The listing builds one solid part. Answer for the finished solid, in the listing's coordinates (mm). Coordinates: 2 decimals unless noted, no trailing zeros. Loops run counter-clockwise (first coordinate to the right, second up) from the corner with the lowest first, then second, coordinate; pieces in that order, holes last. Notation, with made-up numbers: M 24.25,78.25 L 55.25,78.25 A29 cw 55.25,109.25 Z; hole C 61,74 d10. An arc over 180 degrees is marked long. Answer as a JSON object with one key per item and string values. Group by question number.
1. A cutting plane is placed at A-A on y = -127. Give the vertices of the cut face in (x, z).
2. A cutting plane is placed at B-B on z = 3.75. State how many separate pieces and enclosed holes the cut face has, and give its area (3 significant figures).
3. Determine the mould class of faces 1 (the face through (-38.656, -121.646, 6.261)), 2 (the face through (-23.02, -2, 6)), 3 (the face through (-54, 158.75, 6)) for opening direction Y: released by +Y, released by -Y, zero draft, split by the parting line, or undercut.
4. Straight lines are drawn through the part: L1, parallel to X at y = -126.5, z = 3; L2, parallel to X at y = -142, z = 0.75. For each, find the intervals that lie inside material, in ascending order.
from build123d import *

# Parameters (mm, degrees)
F0_R     = 3.96875
F0_R_2   = 6.35
F1_DEPTH = 12.7


with BuildPart() as f1:
    # F0 (on Top) → F1 (new body)
    with BuildSketch(Plane.XY):
        Polygon((-23.019589, 158.75), (-86.519589, 158.75), (-86.519589, -158.75), (-58.071589, -158.75), (-23.019589, -158.75), align=None)
        with Locations((-73.819589, -142.875)):
            Circle(F0_R, mode=Mode.SUBTRACT)
        with Locations((-42.069589, -127)):
            Circle(F0_R_2, mode=Mode.SUBTRACT)
        with Locations((-73.819589, 142.875)):
            Circle(F0_R, mode=Mode.SUBTRACT)
        with Locations((-42.069589, 127)):
            Circle(F0_R_2, mode=Mode.SUBTRACT)
    extrude(amount=F1_DEPTH)


solid = f1.part
From the geometry:
{
 "1": {"outline": "M -86.52,0 L -48.42,0 L -48.42,12.7 L -86.52,12.7 Z; M -35.72,0 L -23.02,0 L -23.02,12.7 L -35.72,12.7 Z"},
 "2": {"separate pieces": "1", "enclosed holes": "4", "area": "19,800 mm²"},
 "3": {"face 1": "undercut", "face 2": "zero draft", "face 3": "released by +Y"},
 "4": {"L1": "x = -86.52 to -48.4, -35.74 to -23.02", "L2": "x = -86.52 to -77.69, -69.95 to -23.02"}
}
